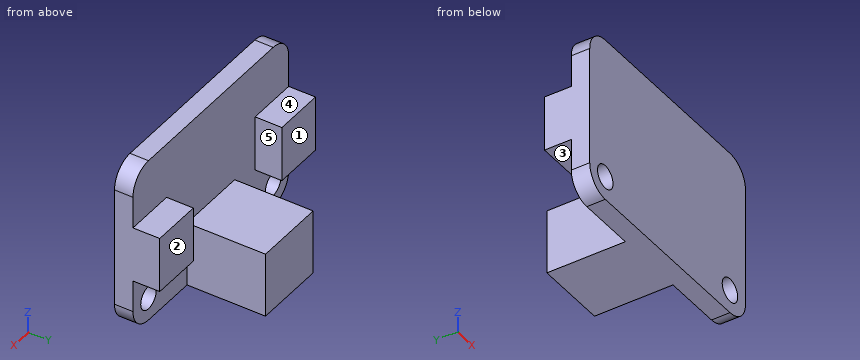
```python
from build123d import *

# Parameters (mm, degrees)
SKETCH1_W           = 25.5
SKETCH1_H           = 18
BOSS_EXTRUDE1_DEPTH = 2
SKETCH2_R           = 1.27
CUT_EXTRUDE1_DEPTH  = 3
SKETCH3_W           = 5.5
SKETCH3_H           = 6
BOSS_EXTRUDE2_DEPTH = 2.9
SKETCH4_W           = 7.8
SKETCH4_H           = 7
BOSS_EXTRUDE3_DEPTH = 8.5
FILLET1_R           = 2.54


with BuildPart() as part:
    # Sketch1 → Boss-Extrude1 (new body)
    with BuildSketch(Plane(origin=(0, 0, 0), x_dir=(1, 0, 0), z_dir=(0, 1, 0))):
        with Locations((12.75, 9)):
            Rectangle(SKETCH1_W, SKETCH1_H)
    extrude(amount=BOSS_EXTRUDE1_DEPTH)

    # Sketch2 → Cut-Extrude1 (cut, through all)
    with BuildSketch(Plane(origin=(0, 2, 0), x_dir=(1, 0, 0), z_dir=(0, 1, 0))):
        with Locations((2.54, 15.46)):
            Circle(SKETCH2_R)
        with Locations((22.96, 15.46)):
            Circle(SKETCH2_R)
    extrude(amount=-CUT_EXTRUDE1_DEPTH, mode=Mode.SUBTRACT)

    # Sketch3 → Boss-Extrude2 (add)
    with BuildSketch(Plane(origin=(0, 2, 0), x_dir=(1, 0, 0), z_dir=(0, 1, 0))):
        with Locations((2.75, 9)):
            Rectangle(SKETCH3_W, SKETCH3_H)
        with Locations((22.75, 9)):
            Rectangle(SKETCH3_W, SKETCH3_H)
    extrude(amount=BOSS_EXTRUDE2_DEPTH)

    # Sketch4 → Boss-Extrude3 (add)
    with BuildSketch(Plane(origin=(0, 2, 0), x_dir=(1, 0, 0), z_dir=(0, 1, 0))):
        with Locations((12.75, 14.5)):
            Rectangle(SKETCH4_W, SKETCH4_H)
    extrude(amount=BOSS_EXTRUDE3_DEPTH)

    # Fillet1
    fillet1_edges = [part.edges().sort_by_distance(p)[0] for p in [
        (0, 1, -18),
        (25.5, 1, -18),
        (25.5, 1, 0),
        (0, 1, 0),
    ]]
    fillet(fillet1_edges, radius=FILLET1_R)


solid = part.part
```
Can you work these out from the model? Positions are in its coordinate system, mm. Face numbers are marked on the shaded views. A direction names the side the tool comes from. Give positions to 0.01 mm unless a question says otherwise; leave off trailing zeros. Loops run counter-clockwise (first coordinate to the right, second up) from the corner with the lowest first, then second, coordinate; pieces in that order, holes last. Notation, with made-up numbers: M 51.5,-35.75 L 82.5,-35.75 A21 ccw 82.5,-5.75 Z; hole C 21.25,87 d3. An arc over 180 degrees is marked long. Use one line per item in the form item = value. Start each with the question number.
(1) I want a section at C-C, the plane x = 12. Write out the boundary of the cut face in (y, z).
(2) I want a section at A-A, the plane y = 4.25. Write out the boundary of the cut face in (x, z), and give its area (3 significant figures).
(3) On a 3-axis mill with a long thin cutter (end or side, diameter ignored), from which of +Z, -Z, +X, -X, +Y, -Y can I reach the whole of each face in a straight line? I mean the marked faces 1, 2, 3, 4 and 5. Say none if no direction works.
(4) I want a section at B-B, the plane z = -10. Write out the boundary of the cut face in (x, y).
(5) I'm going to push flat-ended pins straight in: P1, Ø2, axis at x = 8, y = 7, coming from the +Z side; P2, Ø3, axis at x = 3.5, y = 4, coming from the -Z side; P3, Ø4.5, axis at x = 21.5, z = -10.5, coming from the +Y side; P4, Ø3, axis at y = 8, z = -5.5, coming from the -X side. Where does each tip first touch, or does it pass through?
(6) Please list where these lines run through material, in increasing order: line 1 (X direction, y = 0.65, z = -15.46); line 2 (Z direction, x = 2.54, y = 0.75); line 3 (Z direction, x = 24, y = 4.25).
(7) I want a section at D-D, the plane y = 7. Write out the boundary of the cut face in (x, z).
Worked out:
q1.outline = M 0,-18 L 10.5,-18 L 10.5,-11 L 2,-11 L 2,0 L 0,0 Z
q2.outline = M 0,-12 L 5.5,-12 L 5.5,-6 L 0,-6 Z; M 8.85,-18 L 16.65,-18 L 16.65,-11 L 8.85,-11 Z; M 20,-12 L 25.5,-12 L 25.5,-6 L 20,-6 Z
q2.area = 121 mm²
q3.face_1 = +Z, -Z, -X, +Y
q3.face_2 = +Z, -Z, +X, +Y
q3.face_3 = -Z, -X, +Y
q3.face_4 = +Z, +X, -X, +Y
q3.face_5 = +Z, -Z, +Y
q4.outline = M 0,0 L 25.5,0 L 25.5,4.9 L 20,4.9 L 20,2 L 5.5,2 L 5.5,4.9 L 0,4.9 Z
q5.P1 = -11
q5.P2 = -12
q5.P3 = 4.9
q5.P4 = through
q6.line_1 = 0 to 1.27, 3.81 to 21.69, 24.23 to 25.5
q6.line_2 = -18 to -16.73, -14.19 to 0
q6.line_3 = -12 to -6
q7.outline = M 8.85,-18 L 16.65,-18 L 16.65,-11 L 8.85,-11 Z
